Here's the drawing with two shaded views (mm, measured from the low corner). I have some questions. Coordinates: 2 decimals unless noted, no trailing zeros. Write each loop counter-clockwise with the first axis right and the second up, starting at its lowest first coordinate (ties: lowest second). Pieces come first, ordered by that corner, then holes. Notation, with made-up numbers: (52.5, 61.5) - (67.5, 61.5) arc R22 ccw to (67.5, 98.5) - close; hole circle Ø7 at (-5.5, -27.75). An arc over 180 degrees is marked (long way). Answer in a Markdown table with one row per item. Add a question column.
Item 1: Imagine slicing it at C-C (y = 2.35). Please give me the cut outline in (x, z).
Item 2: Imagine slicing it at B-B (x = 187). Please give me the cut outline in (y, z).
Item 3: If I drill on probe 1 along Z at (x, y) = (12, 2.45); probe 2 along X at (y, z) = (1.95, 12); probe 3 along Z at (x, y) = (9.5, 0.35), over which ranges is the centre line in solid material (lowest first)? Write a range as from..to.
Item 4: Imagine slicing it at A-A (z = 12). Please give me the cut outline in (x, y).
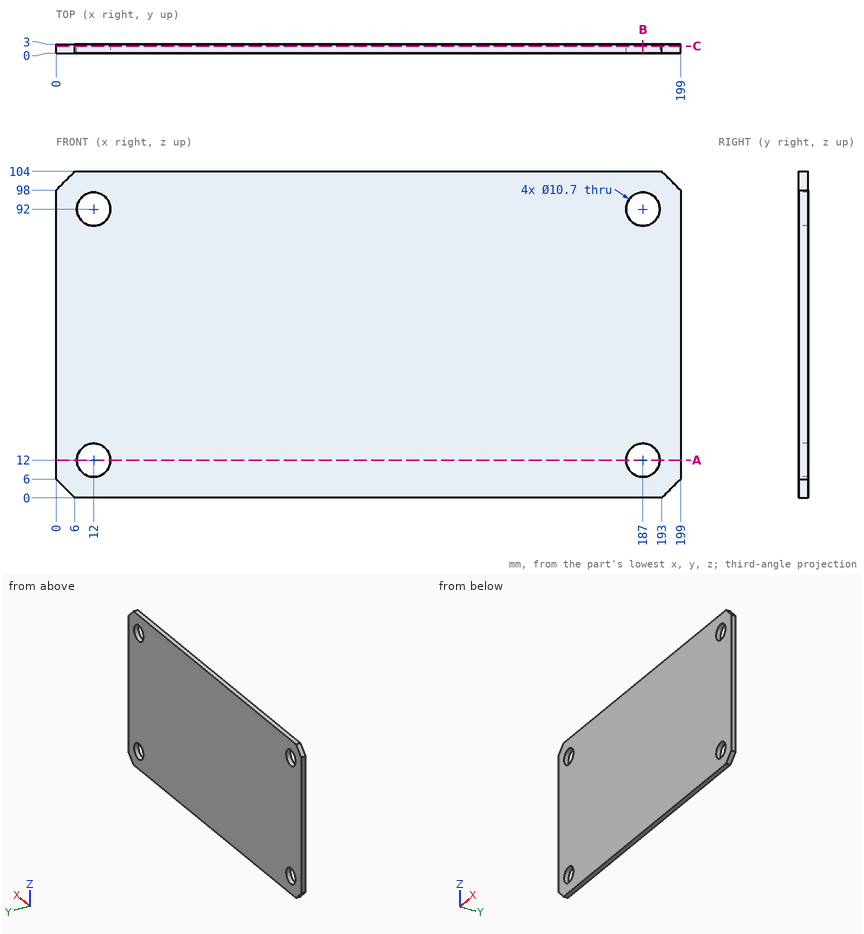
Here are the results:
| question | item | result |
|---|---|---|
| 1 | outline | (0, 6) - (6, 0) - (193, 0) - (199, 6) - (199, 98) - (193, 104) - (6, 104) - (0, 98) - close; hole circle Ø10.7 at (12, 12); hole circle Ø10.7 at (12, 92); hole circle Ø10.7 at (187, 12); hole circle Ø10.7 at (187, 92) |
| 2 | outline | (0, 0) - (3, 0) - (3, 6.65) - (0, 6.65) - close; (0, 17.35) - (3, 17.35) - (3, 86.65) - (0, 86.65) - close; (0, 97.35) - (3, 97.35) - (3, 104) - (0, 104) - close |
| 3 | probe 1 | z = 0..6.65, 17.35..86.65, 97.35..104 |
| 3 | probe 2 | x = 0..6.65, 17.35..181.65, 192.35..199 |
| 3 | probe 3 | z = 0..7.27, 16.73..87.27, 96.73..104 |
| 4 | outline | (0, 0) - (6.65, 0) - (6.65, 3) - (0, 3) - close; (17.35, 0) - (181.65, 0) - (181.65, 3) - (17.35, 3) - close; (192.35, 0) - (199, 0) - (199, 3) - (192.35, 3) - close |
